Work out the finished part from the listing and answer in its coordinate system (mm). A direction names the side the tool comes from. Coordinates: 2 decimals unless noted, no trailing zeros. Loops run counter-clockwise (first coordinate to the right, second up) from the corner with the lowest first, then second, coordinate; pieces in that order, holes last. Notation, with made-up numbers: (67, 62) -> (71, 62) arc R16 ccw to (71, 80) -> close; hole circle Ø7 at (80.25, 18). An arc over 180 degrees is marked (long way). Use a Markdown table: item, result. Add a question column.
```python
from build123d import *

# Parameters (mm, degrees)
SKETCH1_R           = 5.775
BOSS_EXTRUDE1_DEPTH = 10
SKETCH2_R           = 12.7
BOSS_EXTRUDE2_DEPTH = 4.54
SKETCH3_R           = 6.1
BOSS_EXTRUDE3_DEPTH = 4.5
FILLET1_R           = 2


with BuildPart() as part:
    # Sketch1 → Boss-Extrude1 (new body)
    with BuildSketch(Plane(origin=(0, 0, 0), x_dir=(1, 0, 0), z_dir=(0, 1, 0))):
        with Locations(Location((0, 0, 0), (0, 0, 270))):
            Circle(SKETCH1_R)
    extrude(amount=-BOSS_EXTRUDE1_DEPTH)

    # Sketch2 → Boss-Extrude2 (add)
    with BuildSketch(Plane(origin=(0, 0, 0), x_dir=(1, 0, 0), z_dir=(0, 1, 0))):
        with Locations(Location((0, 0, 0), (0, 0, 270))):
            Circle(SKETCH2_R)
    extrude(amount=BOSS_EXTRUDE2_DEPTH)

    # Sketch3 → Boss-Extrude3 (add)
    with BuildSketch(Plane(origin=(0, 4.54, 0), x_dir=(1, 0, 0), z_dir=(0, 1, 0))):
        with Locations(Location((0, 0, 0), (0, 0, 270))):
            Circle(SKETCH3_R)
    extrude(amount=BOSS_EXTRUDE3_DEPTH)

    # Fillet1
    fillet1_edges = [part.edges().sort_by_distance(p)[0] for p in [
        (0, 9.04, -6.1),
    ]]
    fillet(fillet1_edges, radius=FILLET1_R)


solid = part.part
```
Item 1: For faces 1 (the face through (-7.7, 2.2, -10.1)), 2 (the face through (3, 4.54, 5.5)), 3 (the face through (-2.6, 0, 5.5)), determine the directions among +Z, -Z, +X, -X, +Y, -Y from which every point of the face is accessible in a straight line to the end or side of a thin tool.
Item 2: Given pin 1 (2 mm diameter, centred on y = 1, z = 7.5, fed in from -X); pin 2 (2 mm diameter, centred on y = 2, z = -8.5, fed in from -X); pin 3 (5 mm diameter, centred on x = -10, z = 5.5, fed in from -Y); pin 4 (8 mm diameter, centred on x = -6, z = 4.5, fed in from +Y), each flat-ended and moving along its own axis, determine where each tip first touches the part or whether it passes through.
Item 3: Section B-B (z = 0) is taken. Determine the outline of the cut face in (x, y) (3 decimals).
Item 4: Section A-A (x = 0) is taken. Determine the outline of the cut face in (y, z) (3 decimals), then the cut area to 3 significant figures.
Item 5: Section D-D (y = -2) is taken. Determine the outline of the cut face in (x, z) (3 decimals), then the cut area to 3 significant figures.
Item 6: Find the intervals of material crossed by probe 1 along Y at (x, z) = (5, -7); probe 2 along Z at (x, y) = (5.5, 0.25); probe 3 along X at (y, z) = (-4.5, 5.25), in increasing order.
Item 7: Section C-C (y = 6.5) is taken. Determine the outline of the cut face in (x, z).
Output:
| question | item | result |
|---|---|---|
| 1 | face 1 | +Y, -Y |
| 1 | face 2 | +Y |
| 1 | face 3 | -Y |
| 2 | pin 1 | stops at x = -10.91 |
| 2 | pin 2 | stops at x = -10.25 |
| 2 | pin 3 | stops at y = 0 |
| 2 | pin 4 | stops at y = 9.04 |
| 3 | outline | (-12.7, 0) -> (-5.775, 0) -> (-5.775, -10) -> (5.775, -10) -> (5.775, 0) -> (12.7, 0) -> (12.7, 4.54) -> (6.1, 4.54) -> (6.1, 7.04) arc R2 ccw to (4.1, 9.04) -> (-4.1, 9.04) arc R2 ccw to (-6.1, 7.04) -> (-6.1, 4.54) -> (-12.7, 4.54) -> close |
| 4 | outline | (-10, -5.775) -> (0, -5.775) -> (0, -12.7) -> (4.54, -12.7) -> (4.54, -6.1) -> (7.04, -6.1) arc R2 ccw to (9.04, -4.1) -> (9.04, 4.1) arc R2 ccw to (7.04, 6.1) -> (4.54, 6.1) -> (4.54, 12.7) -> (0, 12.7) -> (0, 5.775) -> (-10, 5.775) -> close |
| 4 | area | 284 mm2 |
| 5 | outline | circle Ø11.55 at (0, 0) |
| 5 | area | 105 mm2 |
| 6 | probe 1 | y = 0 to 4.54 |
| 6 | probe 2 | z = -11.45 to 11.45 |
| 6 | probe 3 | x = -2.41 to 2.41 |
| 7 | outline | circle Ø12.2 at (0, 0) |
